from build123d import *

# Parameters (mm, degrees)
F0_R        = 9.8428256451
F0_R_2      = 8.2055899986
F1_DEPTH    = 25.4
F2_DEPTH    = 115.824
F3_DEPTH    = 61.214
F3_FACE_R   = 8.2055899986
F6_S5_R     = 9.8428256451
F6_T6_DEPTH = 20
F5_R        = 7.5988621304
F7_DEPTH    = 107.188
F8_W        = 0.8552042418
F8_H        = 3.9967889898
F8_W_2      = 3.9967889898
F8_H_2      = 0.8552042418
F9_DEPTH    = 6.35


# Not quite as in the source:
# - a fillet or chamfer that OpenCascade refuses, or shapes differently, is made with other operations: its cross-section is extruded or revolved along the edge and cut away or added


with BuildPart() as f1:
    # F0 (on Top) → F1 (new body)
    with BuildSketch(Plane.XY):
        Circle(F0_R)
        Circle(F0_R_2, mode=Mode.SUBTRACT)
    extrude(amount=F1_DEPTH)

    # F2 (add): a face of the model
    f2_faces = [f1.faces().sort_by_distance(p)[0] for p in [
        (-9.5644284947, 0, 0),
    ]]
    extrude(f2_faces, amount=F2_DEPTH)

    # F0 (on Top) → F3 (join)
    with BuildSketch(Plane.XY):
        Circle(F0_R_2)
    extrude(amount=F3_DEPTH)

    # F3_face (on face) → F4 section 0
    with BuildSketch(Plane.XY.offset(61.214), mode=Mode.PRIVATE) as f4_s0:
        Circle(F3_FACE_R)
    loft([Vertex(0, 0, 0), f4_s0.sketch])

    # F6: chamfer of 5.08 on 3 edges, made by hand


with BuildPart() as f6_tool2:
    # F6_s3 → F6_t4 (revolve)
    with BuildSketch(Plane.XZ):
        Polygon((13.2855899986, 25.4), (8.2055899986, 30.48), (8.2055899986, 25.4), align=None)
    revolve(axis=Axis((0, 0, 25.4), (0, 0, 1)))

    # F6_s5 → F6_t6 (intersect, symmetric)
    with BuildSketch(Plane.XY.offset(27.9)):
        Circle(F6_S5_R)
    extrude(amount=F6_T6_DEPTH, both=True, mode=Mode.INTERSECT)


with BuildPart() as f1_1:
    add(f1.part)

    # F6_t1: union F6_tool2
    add(f6_tool2.part)

    # F6_s7 → F6_t8 (revolve, cut)
    with BuildSketch(Plane.XZ):
        Polygon((8.2055899986, 56.134), (3.1255899986, 61.214), (8.2055899986, 61.214), align=None)
    revolve(axis=Axis((0, 0, 61.214), (0, 0, 1)), mode=Mode.SUBTRACT)

    # F5 (on Top) → F7 (join)
    with BuildSketch(Plane.XY):
        Circle(F5_R)
    extrude(amount=-F7_DEPTH)

    # F8 (on face) → F9 (join)
    with BuildSketch(Plane(origin=(0, 0, -107.188), x_dir=(1, 0, 0), z_dir=(0, 0, -1))):
        with Locations((0.0061568862, 6.3575312961)):
            Rectangle(F8_W, F8_H)
        Polygon((-6.2065385732, 5.6105250065), (-3.3803819756, 2.7843684089), (-2.7756612569, 3.3890891276), (-5.6018178545, 6.2152457252), align=None)
        with Locations((-6.3575312961, 0.0061568862)):
            Rectangle(F8_W_2, F8_H_2)
        Polygon((-5.6105250065, -6.2065385732), (-2.7843684089, -3.3803819756), (-3.3890891276, -2.7756612569), (-6.2152457252, -5.6018178545), align=None)
        with Locations((-0.0061568862, -6.3575312961)):
            Rectangle(F8_W, F8_H)
        Polygon((6.2065385732, -5.6105250065), (3.3803819756, -2.7843684089), (2.7756612569, -3.3890891276), (5.6018178545, -6.2152457252), align=None)
        with Locations((6.3575312961, -0.0061568862)):
            Rectangle(F8_W_2, F8_H_2)
        Polygon((5.6105250065, 6.2065385732), (2.7843684089, 3.3803819756), (3.3890891276, 2.7756612569), (6.2152457252, 5.6018178545), align=None)
    extrude(amount=F9_DEPTH)


solid = f1_1.part
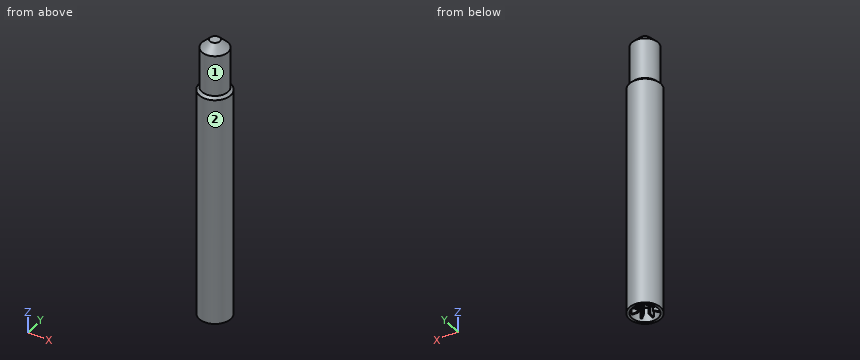
Verification items for the finished model (mm, model axes). Face numbers are marked on the shaded views. A direction names the side the tool comes from. Coordinates: 2 decimals unless noted, no trailing zeros. Write each loop counter-clockwise with the first axis right and the second up, starting at its lowest first coordinate (ties: lowest second). Pieces come first, ordered by that corner, then holes. Notation, with made-up numbers: (87, 56.5) - (128, 56.5) arc R23 cw to (128, 89.5) - close; hole circle Ø8 at (26, -4). An arc over 180 degrees is marked (long way). Answer as a JSON object with one key per item and string values.
(1) Thickness scan on line 1 along Y through (x, z) = (0, -40.5); line 2 along Y through (x, z) = (7, -41.5); line 3 along X through (y, z) = (-0.25, -70). Record the ranges inside material, lowest first.
Report:
{"line 1": "-9.84 to -8.21, -7.6 to 7.6, 8.21 to 9.84", "line 2": "-6.92 to -4.28, -2.96 to 2.96, 4.28 to 6.92", "line 3": "-9.84 to -8.2, -7.59 to 7.59, 8.2 to 9.84"}
(2) Tool access check on the marked faces 1 and 2. Record the directions out of +Z, -Z, +X, -X, +Y, -Y that give a thin tool (end or side, any length) a straight path to the whole face; none if there is none.
Report:
{"face 1": "+Z", "face 2": "+Z, -Z"}
(3) Gauge pin test, flat ends, axial feed: pin 1 Ø1.9 at (y, z) = (6.5, -110) entering from +X; pin 2 Ø4 at (x, y) = (-6, -5) entering from +Z; pin 3 Ø0.5 at (x, y) = (-5.5, 6) entering from +Z. Record the tip position at first contact, or that the pin passes through.
Report:
{"pin 1": "x = 8.13", "pin 2": "z = 58.53", "pin 3": "z = 56.45"}
(4) Cross-section at A-A on z = -65.5. Record the cut outline in (x, y), plus the area to 3 significant figures.
Report:
{"outline": "circle Ø19.69 at (0, 0); circle Ø15.2 at (0, 0); hole circle Ø16.41 at (0, 0)", "area": "274 mm^2"}
(5) Cross-section at B-B on z = 50. Record the cut outline in (x, y).
Report:
{"outline": "circle Ø16.41 at (0, 0)"}
